```python
from build123d import *

# Parameters (mm, degrees)
ESQUISSE1_W              = 105
ESQUISSE1_H              = 80
BOSS_EXTRU_1_DEPTH       = 25
ESQUISSE2_R              = 7.9
ESQUISSE2_R_2            = 7.95
ESQUISSE2_R_3            = 4.5
ENL_V_MAT_EXTRU_1_DEPTH  = 135.350288425
ESQUISSE3_R              = 4
ENL_V_MAT_EXTRU_3_DEPTH  = 10
ESQUISSE6_W              = 40
ESQUISSE6_H              = 80
ENL_V_MAT_EXTRU_6_DEPTH  = 135.350288425
ESQUISSE7_W              = 65
ESQUISSE7_H              = 2.68813313
ENL_V_MAT_EXTRU_7_DEPTH  = 135.350288425
CONG_1_R                 = 3
ESQUISSE9_W              = 5
ESQUISSE9_H              = 20.179429856
ESQUISSE9_H_2            = 20.18
BOSS_EXTRU_2_DEPTH       = 25
ESQUISSE10_R             = 2.5
ENL_V_MAT_EXTRU_8_DEPTH  = 105.048287139
ENL_V_MAT_EXTRU_9_DEPTH  = 7.5
ENL_V_MAT_EXTRU_11_DEPTH = 133.767182537
ESQUISSE13_R             = 1.5
ENL_V_MAT_EXTRU_12_DEPTH = 3


with BuildPart() as part:
    # Esquisse1 → Boss.-Extru.1 (new body)
    with BuildSketch(Plane.XY):
        with Locations((52.5, 40)):
            Rectangle(ESQUISSE1_W, ESQUISSE1_H)
    extrude(amount=BOSS_EXTRU_1_DEPTH)

    # Esquisse2 → Enlèv. mat.-Extru.1 (cut, through all)
    with BuildSketch(Plane.XY):
        with Locations((63.7, 10)):
            Circle(ESQUISSE2_R)
        with Locations((80, 10)):
            Circle(ESQUISSE2_R_2)
        with Locations((71.85, 24.633523157)):
            Circle(ESQUISSE2_R_3)
    extrude(amount=ENL_V_MAT_EXTRU_1_DEPTH, mode=Mode.SUBTRACT)

    # Esquisse3 → Enlèv. mat.-Extru.3 (cut)
    with BuildSketch(Plane(origin=(0, 0, 0), x_dir=(1, 0, 0), z_dir=(0, 1, 0))):
        with Locations(Location((49, -12.5, 0), (0, 0, 270))):
            Circle(ESQUISSE3_R)
        with Locations(Location((93, -12.5, 0), (0, 0, 270))):
            Circle(ESQUISSE3_R)
    extrude(amount=ENL_V_MAT_EXTRU_3_DEPTH, mode=Mode.SUBTRACT)

    # Esquisse6 → Enlèv. mat.-Extru.6 (cut, through all)
    with BuildSketch(Plane.XY):
        with Locations((20, 40)):
            Rectangle(ESQUISSE6_W, ESQUISSE6_H)
    extrude(amount=ENL_V_MAT_EXTRU_6_DEPTH, mode=Mode.SUBTRACT)

    # Esquisse7 → Enlèv. mat.-Extru.7 (cut, through all)
    with BuildSketch(Plane.XY):
        with Locations((72.5, 78.655933435)):
            Rectangle(ESQUISSE7_W, ESQUISSE7_H)
    extrude(amount=ENL_V_MAT_EXTRU_7_DEPTH, mode=Mode.SUBTRACT)

    # Congé1
    cong_1_edges = [part.edges().sort_by_distance(p)[0] for p in [
        (40, 0, 12.5),
        (105, 77.31186687, 12.5),
        (40, 77.31186687, 12.5),
        (105, 0, 12.5),
    ]]
    fillet(cong_1_edges, radius=CONG_1_R)

    # Esquisse9 → Boss.-Extru.2 (add)
    with BuildSketch(Plane.XY):
        with Locations((102.49170176, 42.222151942)):
            Rectangle(ESQUISSE9_W, ESQUISSE9_H)
        with Locations((80.49170176, 42.22186687)):
            Rectangle(ESQUISSE9_W, ESQUISSE9_H_2)
    extrude(amount=-BOSS_EXTRU_2_DEPTH)

    # Esquisse10 → Enlèv. mat.-Extru.8 (cut, through all)
    with BuildSketch(Plane(origin=(104.99170176, 0, 0), x_dir=(0, 0, -1), z_dir=(1, 0, 0))):
        with Locations((21.24, 42.132437014)):
            Circle(ESQUISSE10_R)
    extrude(amount=-ENL_V_MAT_EXTRU_8_DEPTH, mode=Mode.SUBTRACT)

    # Esquisse11 → Enlèv. mat.-Extru.9 (cut)
    with BuildSketch(Plane(origin=(0, 0, 0), x_dir=(-1, 0, 0), z_dir=(0, 0, -1))):
        Polygon((-73.38169787, 32.15796566), (-79.132207291, 27.069255143), (-77.600509422, 19.54481264), (-70.31830213, 17.109080655), (-64.567792709, 22.197791172), (-66.099490578, 29.722233675), align=None)
    extrude(amount=-ENL_V_MAT_EXTRU_9_DEPTH, mode=Mode.SUBTRACT)

    # Esquisse12 → Enlèv. mat.-Extru.11 (cut, through all)
    with BuildSketch(Plane(origin=(0, 0, 0), x_dir=(-1, 0, 0), z_dir=(0, 0, -1))):
        Polygon((-105.676011247, 77.330619324), (-105.676011247, 52.31186687), (-104.99170176, 52.31186687), (-39.98533212, 52.31186687), (-39.98533212, 77.330619324), (-104.99170176, 77.330619324), align=None)
    extrude(amount=-ENL_V_MAT_EXTRU_11_DEPTH, mode=Mode.SUBTRACT)

    # Esquisse13 → Enlèv. mat.-Extru.12 (cut)
    with BuildSketch(Plane.ZY.offset(-40)):
        with Locations((15, 14.75187619)):
            Circle(ESQUISSE13_R)
        with Locations((15, 26)):
            Circle(ESQUISSE13_R)
    extrude(amount=-ENL_V_MAT_EXTRU_12_DEPTH, mode=Mode.SUBTRACT)


solid = part.part
```
Work out the finished part from the listing and answer in its coordinate system (mm). A direction names the side the tool comes from. Round coordinates to 2 decimals unless told otherwise and drop trailing zeros. Loops run counter-clockwise (first coordinate to the right, second up) from the corner with the lowest first, then second, coordinate; pieces in that order, holes last. Notation, with made-up numbers: M 39.5,48.25 L 91.5,48.25 A27 ccw 91.5,73.25 Z; hole C -29.75,22 d9. An arc over 180 degrees is marked long. One line per question, with ' | ' between items.
Q1. Consider line 1 along X through (y, z) = (10, 18); line 2 along X through (y, z) = (11.5, 3); line 3 along X through (y, z) = (40, -5). Determine where each line is inside the solid, lowest interval first. Write a range as from..to.
Conclusion:
line 1: x = 40..55.8, 71.6..72.05, 87.95..105 | line 2: x = 40..55.94, 71.46..72.19, 87.81..105 | line 3: x = 77.99..82.99, 99.99..104.99
Q2. Find section A-A, the plane x = 63.7. Give the vertices of the cut face in (y, z).
Conclusion:
outline: M 0,0 L 2.1,0 L 2.1,25 L 0,25 Z; M 17.9,0 L 52.31,0 L 52.31,25 L 17.9,25 Z
Q3. A tool of negligible diameter and unlimited length cuts with its end or side. For faces 4 (the flat face through (82.992, 42, -12)), 5 (the flat face through (93, 10, 12)), 6 (the flat face through (67.48, 19.62, 3.7)), 7 (the flat face through (80, 32.132, -12)), 8 (the flat face through (77.992, 42, -12)), from which of +Z, -Z, +X, -X, +Y, -Y can it reach the whole face along a straight path? Write none if from no direction.
Conclusion:
face 4: -Z, +Y, -Y | face 5: -Y | face 6: -Z | face 7: -Z, +X, -X, -Y | face 8: -Z, -X, +Y, -Y
Q4. Each of these flat-tipped pins is pushed along its axis until it touches: pin 1 Ø4 at (x, z) = (49, 13.5) entering from -Y; pin 2 Ø6.5 at (y, z) = (42.13, -21.24) entering from -X; pin 3 Ø2.5 at (y, z) = (26, 15) entering from -X; pin 4 Ø10.5 at (x, z) = (93, 12.5) entering from -Y. Where does it stop, or does it pass through?
Conclusion:
pin 1: stops at y = 10 | pin 2: stops at x = 77.99 | pin 3: stops at x = 43 | pin 4: stops at y = 0
Q5. Find section C-C, the plane z = -14.5. Give the vertices of the cut face in (x, y), then the cut area to 3 significant figures.
Conclusion:
outline: M 77.99,32.13 L 82.99,32.13 L 82.99,52.31 L 77.99,52.31 Z; M 99.99,32.13 L 104.99,32.13 L 104.99,52.31 L 99.99,52.31 Z | area: 202 mm2
Q6. The mould has two halves that part along Z. Classify faces 1 (the flat face through (72, 32, 25)), 2 (the cylindrical face through (41.48, 27.01, 13.89)), 3 (the flat face through (102, 32.132, -12)): +Z half, -Z half, draft (parallel to the pull), parting line (faces both ways), or undercut.
Conclusion:
face 1: +Z half | face 2: undercut | face 3: draft
Q7. Find section B-B, the plane z = -21.24. Give the vertices of the cut face in (x, y).
Conclusion:
outline: M 77.99,32.13 L 82.99,32.13 L 82.99,39.63 L 77.99,39.63 Z; M 77.99,44.63 L 82.99,44.63 L 82.99,52.31 L 77.99,52.31 Z; M 99.99,32.13 L 104.99,32.13 L 104.99,39.63 L 99.99,39.63 Z; M 99.99,44.63 L 104.99,44.63 L 104.99,52.31 L 99.99,52.31 Z
Q8. Find section D-D, the plane x = 93. Give the vertices of the cut face in (y, z).
Conclusion:
outline: M 0,0 L 52.31,0 L 52.31,25 L 0,25 L 0,16.5 L 10,16.5 L 10,8.5 L 0,8.5 Z
